from build123d import *

# Parameters (mm, degrees)
SKETCH1_W          = 101.6
SKETCH1_H          = 101.6
EXTRUDE1_DEPTH     = 79.502
SKETCH2_R          = 33.401
EXTRUDE2_DEPTH     = 9.398
CHAMFER1_SIZE      = 1.524
SKETCH3_R          = 13.4874
CUT_EXTRUDE1_DEPTH = 89.9
SKETCH4_R          = 5.5499
CUT_EXTRUDE2_DEPTH = 12.7
HOLE1_D            = 7.9375
HOLE1_DEPTH        = 12.7


with BuildPart() as part:
    # Sketch1 → Extrude1 (new body)
    with BuildSketch(Plane(origin=(0, 0, 0), x_dir=(1, 0, 0), z_dir=(0, 1, 0))):
        Rectangle(SKETCH1_W, SKETCH1_H)
    extrude(amount=EXTRUDE1_DEPTH)

    # Sketch2 → Extrude2 (add)
    with BuildSketch(Plane(origin=(0, 79.502, 0), x_dir=(-1, 0, 0), z_dir=(0, 1, 0))):
        with Locations(Location((0, 0, 0), (0, 0, 90))):  # turned: the seam where the file's is
            Circle(SKETCH2_R)
    extrude(amount=EXTRUDE2_DEPTH)

    # Chamfer1
    chamfer1_edges = [part.edges().sort_by_distance(p)[0] for p in [
        (0, 88.9, -33.401),
    ]]
    chamfer(chamfer1_edges, length=CHAMFER1_SIZE)

    # Sketch3 → Cut-Extrude1 (cut, through all)
    with BuildSketch(Plane(origin=(0, 88.9, 0), x_dir=(1, 0, 0), z_dir=(0, 1, 0))):
        with Locations(Location((0, 0, 0), (0, 0, 270))):  # turned: the seam where the file's is
            Circle(SKETCH3_R)
    extrude(amount=-CUT_EXTRUDE1_DEPTH, mode=Mode.SUBTRACT)

    # Sketch4 → Cut-Extrude2 (cut)
    with BuildSketch(Plane.XY.offset(50.8)):
        with Locations((0, 69.85)):
            Circle(SKETCH4_R)
        with Locations((0, 12.7)):
            Circle(SKETCH4_R)
    extrude(amount=-CUT_EXTRUDE2_DEPTH, mode=Mode.SUBTRACT)

    # Hole1
    with Locations(Plane.XZ):
        with Locations((-38.1, 38.1), (38.1, 38.1), (38.1, -38.1), (-38.1, -38.1)):
            Hole(HOLE1_D / 2, depth=HOLE1_DEPTH)


solid = part.part
The listing builds one solid part. Answer for the finished solid, in the listing's coordinates (mm). A direction names the side the tool comes from. Give positions to 0.01 mm unless a question says otherwise; leave off trailing zeros. Order: outer loops, then holes, each group sorted by start corner. A loop starts at its lowest first (then second) coordinate and runs counter-clockwise, first axis right, second up. Notation, with made-up numbers: (-0.75, 52) - (37.25, 52) arc R19 cw to (37.25, 66) - close; hole circle Ø1 at (-7.5, 70.25). An arc over 180 degrees is marked (long way). Answer as CSV lines item,"result".
Q1. A cutting plane is placed at B-B, the plane z = 0. Determine the outline of the cut face in (x, y).
Answer key:
outline,"(-50.8, 0) - (-13.49, 0) - (-13.49, 88.9) - (-31.88, 88.9) - (-33.4, 87.38) - (-33.4, 79.5) - (-50.8, 79.5) - close; (13.49, 0) - (50.8, 0) - (50.8, 79.5) - (33.4, 79.5) - (33.4, 87.38) - (31.88, 88.9) - (13.49, 88.9) - close"
Q2. Determine the mould class of faces 6 (the face through (38, 12.7, -38)), 7 (the face through (-32.607, 83.384, -7.241)), 8 (the face through (50.8, 39, 1)), 9 (the face through (0, 88.9, 14)) for opening direction X: pulls with the +X half, pulls with the -X half, needs draft (parallel to the pull), parting line crosses it, or undercut.
Answer key:
face 6,"undercut"
face 7,"parting line crosses it"
face 8,"pulls with the +X half"
face 9,"needs draft"
Q3. Each of these flat-tipped pins is pushed along its axis until it touches: pin 1 Ø2.5 at (x, z) = (38.5, -38.5) entering from -Y; pin 2 Ø5.5 at (x, y) = (0.5, 15) entering from +Z; pin 3 Ø7 at (x, z) = (38.1, -38.1) entering from +Y. Where does it stop, or does it pass through?
Answer key:
pin 1,"stops at y = 12.7"
pin 2,"stops at z = 38.1"
pin 3,"stops at y = 79.5"
Q4. A cutting plane is placed at D-D, the plane y = 69.85. Determine the outline of the cut face in (x, z), and give its area (3 significant figures).
Answer key:
outline,"(-50.8, -50.8) - (50.8, -50.8) - (50.8, 50.8) - (5.55, 50.8) - (5.55, 38.1) - (-5.55, 38.1) - (-5.55, 50.8) - (-50.8, 50.8) - close; hole circle Ø26.97 at (0, 0)"
area,"9,610 mm^2"
Q5. Straight lines are drawn through the part: L1, parallel to Z at x = 38.1, y = 8.5; L2, parallel to Y at x = 0, z = 45.5. For each, find the intervals that lie inside material, in ascending order.
Answer key:
L1,"z = -50.8 to -42.07, -34.13 to 34.13, 42.07 to 50.8"
L2,"y = 0 to 7.15, 18.25 to 64.3, 75.4 to 79.5"
Q6. Which of the six approach directions +Z, -Z, +X, -X, +Y, -Y give full straight-line access (tool end or side, diameter ignored) to faces 1 (the face through (0, 13, 38.1)), 2 (the face through (11, 0, -12)), 3 (the face through (-1, 39, 50.8)), 4 (the face through (-38, 12.7, -38)), 5 (the face through (-1, 79.502, -35))?
Answer key:
face 1,"+Z"
face 2,"+Z, -Z, +X, -X, -Y"
face 3,"+Z, +X, -X, +Y, -Y"
face 4,"-Y"
face 5,"+Y"
Q7. A cutting plane is placed at A-A, the plane y = 5. Determine the outline of the cut face in (x, z).
Answer key:
outline,"(-50.8, -50.8) - (50.8, -50.8) - (50.8, 50.8) - (-50.8, 50.8) - close; hole circle Ø7.94 at (-38.1, -38.1); hole circle Ø7.94 at (-38.1, 38.1); hole circle Ø26.97 at (0, 0); hole circle Ø7.94 at (38.1, -38.1); hole circle Ø7.94 at (38.1, 38.1)"
Q8. A cutting plane is placed at C-C, the plane x = 0. Determine the outline of the cut face in (y, z).
Answer key:
outline,"(0, -50.8) - (79.5, -50.8) - (79.5, -33.4) - (87.38, -33.4) - (88.9, -31.88) - (88.9, -13.49) - (0, -13.49) - close; (0, 13.49) - (88.9, 13.49) - (88.9, 31.88) - (87.38, 33.4) - (79.5, 33.4) - (79.5, 50.8) - (75.4, 50.8) - (75.4, 38.1) - (64.3, 38.1) - (64.3, 50.8) - (18.25, 50.8) - (18.25, 38.1) - (7.15, 38.1) - (7.15, 50.8) - (0, 50.8) - close"
